Source: CAD feature listing. Evaluate the final solid. Frame: model axes, mm. Face numbers are marked on the shaded views. A direction names the side the tool comes from. Round coordinates to 2 decimals unless told otherwise and drop trailing zeros. Loops run counter-clockwise (first coordinate to the right, second up) from the corner with the lowest first, then second, coordinate; pieces in that order, holes last. Notation, with made-up numbers: (-8.75, 36) -> (32.25, 36) arc R9 ccw to (32.25, 42) -> close; hole circle Ø11 at (-23.75, 32.25). An arc over 180 degrees is marked (long way). Put each result on its own line as item: value. Start each with the question number.
1. Set-up query: the marked faces 4, 5, 6 and 7. Return all of +Z, -Z, +X, -X, +Y, -Y with unobstructed straight access to the full face (end or side cutting, diameter ignored); none if empty.
2. Cut plane A-A (z = 45). Return the cut outline in (x, y), then the cut area to 3 significant figures.
3. Draft query along Y for the marked faces 1, 2 and 3. Return one class per face: pulls with the +Y half, pulls with the -Y half, needs draft (parallel to the pull), parting line crosses it, or undercut.
4. Contact query for flat-ended pins moving along their axis: pin 1 (1 mm diameter, centred on x = -11, z = 19.5, fed in from -Y); pin 2 (13.5 mm diameter, centred on x = -82, z = 83, fed in from +Y); pin 3 (12 mm diameter, centred on y = 34, z = 35.5, fed in from +X). Output: stop coordinate, or through.
5. Material intervals for L1, parallel to Y at x = 0, z = 70; L2, parallel to X at y = 57, z = 95; L3, parallel to Y at x = 7, z = 115.5, sorted ascending.
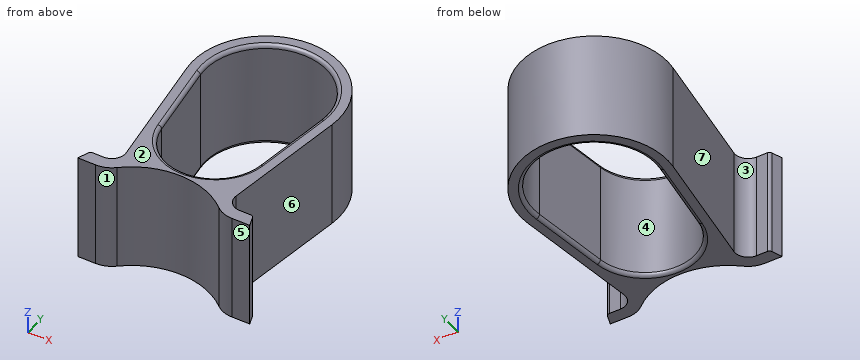
```python
from build123d import *

# Parameters (mm, degrees)
PAD_DEPTH = 120
FILLET_R  = 4


with BuildPart() as part:
    # Sketch → Pad (new body)
    with BuildSketch(Plane.XY):
        with BuildLine():
            ThreePointArc((81.205589, 163.61348), (0, 257.000003), (-81.205589, 163.61348))
            Line((-61.604046, 23.818887), (-81.205589, 163.61348))
            ThreePointArc((-76.312668, 7.000001), (-65.141069, 12.071111), (-61.604046, 23.818887))
            Line((-76.312668, 7.000001), (-91.312668, 7.000001))
            Line((-91.312668, 7.000001), (-96.311409, -6.989133))
            Line((-76.311409, -6.989133), (-96.311409, -6.989133))
            ThreePointArc((-76.311409, -6.989133), (-66.118961, -5.12685), (-57.243123, 0.218577))
            ThreePointArc((57.192961, 0.198819), (-0.021346, 21.841028), (-57.243123, 0.218577))
            ThreePointArc((57.192961, 0.198819), (66.053148, -5.140178), (76.229044, -6.999999))
            Line((76.229044, -6.999999), (96.229044, -6.999999))
            Line((91.229042, 7.000001), (96.229044, -6.999999))
            Line((76.229042, 7.000001), (91.229042, 7.000001))
            ThreePointArc((61.603815, 23.818922), (65.084835, 12.077624), (76.229042, 7.000001))
            Line((81.205589, 163.61348), (61.603815, 23.818922))
        make_face()
        with BuildLine():
            ThreePointArc((67.341217, 165.557526), (0, 243.000004), (-67.341217, 165.557526))
            Line((-67.341217, 165.557526), (-54.868226, 76.553143))
            ThreePointArc((-54.868226, 76.553143), (-0.005687, 28.841012), (54.860565, 76.548873))
            Line((67.341217, 165.557526), (54.860565, 76.548873))
        make_face(mode=Mode.SUBTRACT)
    extrude(amount=PAD_DEPTH)

    # Fillet
    fillet_edges = [part.edges().sort_by_distance(p)[0] for p in [
        (-54.868226, 76.553143, 60),
        (54.860565, 76.548873, 60),
        (-0.005687, 28.841012, 0),
        (-0.005687, 28.841012, 120),
        (-67.341217, 165.557526, 60),
        (-61.104722, 121.055334, 0),
        (-61.104722, 121.055334, 120),
        (67.341217, 165.557526, 60),
        (0, 243.000004, 0),
        (0, 243.000004, 120),
        (61.100891, 121.0532, 0),
        (61.100891, 121.0532, 120),
        (-91.312668, 7.000001, 60),
        (91.229042, 7.000001, 60),
    ]]
    fillet(fillet_edges, radius=FILLET_R)


solid = part.part
```
Solution:
1. face 4: +Z, -Z
1. face 5: +Z, -Z, +X, -X, -Y
1. face 6: +Z, -Z, +X
1. face 7: +Z, -Z, -X
2. outline: (-96.31, -6.99) -> (-76.31, -6.99) arc R28.83 ccw to (-57.24, 0.22) arc R86.49 cw to (57.19, 0.2) arc R28.77 ccw to (76.23, -7) -> (96.23, -7) -> (92.18, 4.35) arc R4 ccw to (88.41, 7) -> (76.23, 7) arc R14.77 cw to (61.6, 23.82) -> (81.21, 163.61) arc R82 ccw (long way) to (-81.21, 163.61) -> (-61.6, 23.82) arc R14.84 cw to (-76.31, 7) -> (-88.49, 7) arc R4 ccw to (-92.26, 4.35) -> close; hole (-67.34, 165.56) -> (-54.87, 76.55) arc R55.4 ccw to (54.86, 76.55) -> (67.34, 165.56) arc R68 ccw (long way) to start
2. area: 11,200 mm^2
3. face 1: pulls with the -Y half
3. face 2: needs draft
3. face 3: undercut
4. pin 1: stops at y = 21.08
4. pin 2: stops at y = 207.58
4. pin 3: stops at x = 63.87
5. L1: y = 21.84 to 28.84, 243 to 257
5. L2: x = -66.26 to -48.24, 48.24 to 66.26
5. L3: y = 21.55 to 29.29, 242.64 to 256.7
